```python
from build123d import *

# Parameters (mm, degrees)
ESQUISSE1_W             = 19.5
ESQUISSE1_H             = 1.5
EXTRU_MINCE1_DEPTH      = 96
ESQUISSE2_W             = 1.5
ESQUISSE2_H             = 19.5
EXTRU_MINCE2_DEPTH      = 96
ESQUISSE3_R             = 1.5
ESQUISSE3_W             = 18
ESQUISSE3_H             = 18
ENL_V_MAT_EXTRU_1_DEPTH = 3
ESQUISSE4_R             = 2
ESQUISSE4_R_2           = 1.5
ESQUISSE4_W             = 5
ESQUISSE4_H             = 20
ENL_V_MAT_EXTRU_2_DEPTH = 3
CONG_1_R                = 4


with BuildPart() as part:
    # Esquisse1 → Extru.-Mince1 (new body)
    with BuildSketch(Plane.XY):
        with Locations((0, 0.75)):
            Rectangle(ESQUISSE1_W, ESQUISSE1_H)
    extrude(amount=EXTRU_MINCE1_DEPTH)

    # Esquisse2 → Extru.-Mince2 (add)
    with BuildSketch(Plane(origin=(0, 0, 0), x_dir=(-1, 0, 0), z_dir=(0, 0, -1))):
        with Locations((0, 9.75)):
            Rectangle(ESQUISSE2_W, ESQUISSE2_H)
    extrude(amount=-EXTRU_MINCE2_DEPTH)

    # Esquisse3 → Enlèv. mat.-Extru.1 (cut)
    with BuildSketch(Plane.ZY.offset(0.75)):
        with Locations((48, 16)):
            Circle(ESQUISSE3_R)
        with Locations((9, 10.5)):
            Rectangle(ESQUISSE3_W, ESQUISSE3_H)
        with Locations((87, 10.5)):
            Rectangle(ESQUISSE3_W, ESQUISSE3_H)
    extrude(amount=-ENL_V_MAT_EXTRU_1_DEPTH, mode=Mode.SUBTRACT)

    # Esquisse4 → Enlèv. mat.-Extru.2 (cut)
    with BuildSketch(Plane(origin=(0, 1.5, 0), x_dir=(1, 0, 0), z_dir=(0, 1, 0))):
        with Locations(Location((-0.75, -10, 0), (0, 0, 270))):
            Circle(ESQUISSE4_R)
        with Locations(Location((-0.75, -86, 0), (0, 0, 270))):
            Circle(ESQUISSE4_R)
        with Locations(Location((6.75, -48, 0), (0, 0, 270))):
            Circle(ESQUISSE4_R_2)
        with Locations((7.25, -86)):
            Rectangle(ESQUISSE4_W, ESQUISSE4_H)
    extrude(amount=-ENL_V_MAT_EXTRU_2_DEPTH, mode=Mode.SUBTRACT)

    # Congé1
    cong_1_edges = [part.edges().sort_by_distance(p)[0] for p in [
        (4.75, 0.75, 76),
    ]]
    fillet(cong_1_edges, radius=CONG_1_R)


solid = part.part
```
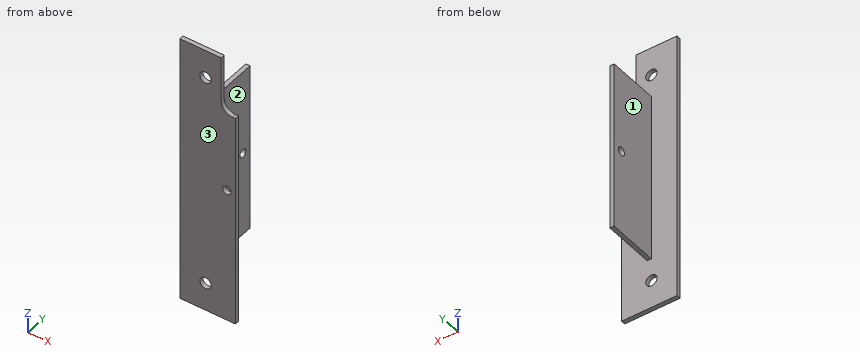
Model file for the job. Use its own axes, mm. Face numbers are marked on the shaded views. A direction names the side the tool comes from. Coordinates: 2 decimals unless noted, no trailing zeros. Write each loop counter-clockwise with the first axis right and the second up, starting at its lowest first coordinate (ties: lowest second). Pieces come first, ordered by that corner, then holes. Notation, with made-up numbers: (62, -23.75) - (77, -23.75) arc R22 ccw to (77, 3.25) - close; hole circle Ø1 at (64, 69.5). An arc over 180 degrees is marked (long way). Use a Markdown table: item, result. Add a question column.
Item 1: Band-saw the part on D-D, the plane z = 38. Write the cut outline in (x, y).
Item 2: 3-axis set-ups, long thin cutter, end or side, ignore diameter. For the marked faces 1, 2 and 3: which of +Z, -Z, +X, -X, +Y, -Y reach the whole face in a straight line?
Item 3: Drill centre lines: line 1 along X through (y, z) = (1.25, 10); line 2 along Y through (x, z) = (0.1, 48); line 3 along Y through (x, z) = (4.75, 72). Where is each one in solid material? Low to high.
Item 4: Band-saw the part on B-B, the plane y = 16. Write the cut outline in (x, z).
Item 5: Drop flat-ended pins along their axis: pin 1 (1 mm diameter, centred on x = -0.5, y = 6.5, fed in from -Z); pin 2 (6 mm diameter, centred on y = 16, z = 41.5, fed in from +X); pin 3 (6.5 mm diameter, centred on x = -0.75, z = 10, fed in from +Y). Give the stop position or say it passes through.
Item 6: Band-saw the part on C-C, the plane z = 48. Write the cut outline in (x, y), and give its area (4 significant figures).
Item 7: Band-saw the part on A-A, the plane z = 86. Write the cut outline in (x, y).
A:
| question | item | result |
|---|---|---|
| 1 | outline | (-9.75, 0) - (9.75, 0) - (9.75, 1.5) - (0.75, 1.5) - (0.75, 19.5) - (-0.75, 19.5) - (-0.75, 1.5) - (-9.75, 1.5) - close |
| 2 | face 1 | +Z, -Z, -X, +Y |
| 2 | face 2 | +Z, -Z, +X, +Y |
| 2 | face 3 | +Z, -Z, +X, -X, -Y |
| 3 | line 1 | x = -9.75 to -2.75, 1.25 to 9.75 |
| 3 | line 2 | y = 0 to 14.5, 17.5 to 19.5 |
| 3 | line 3 | y = 0 to 1.5 |
| 4 | outline | (-0.75, 18) - (0.75, 18) - (0.75, 46.5) - (-0.75, 46.5) - close; (-0.75, 49.5) - (0.75, 49.5) - (0.75, 78) - (-0.75, 78) - close |
| 5 | pin 1 | stops at z = 18 |
| 5 | pin 2 | stops at x = 0.75 |
| 5 | pin 3 | stops at y = 1.5 |
| 6 | outline | (-9.75, 0) - (5.25, 0) - (5.25, 1.5) - (0.75, 1.5) - (0.75, 14.5) - (-0.75, 14.5) - (-0.75, 1.5) - (-9.75, 1.5) - close; (-0.75, 17.5) - (0.75, 17.5) - (0.75, 19.5) - (-0.75, 19.5) - close; (8.25, 0) - (9.75, 0) - (9.75, 1.5) - (8.25, 1.5) - close |
| 6 | area | 47.25 mm² |
| 7 | outline | (-9.75, 0) - (-2.75, 0) - (-2.75, 1.5) - (-9.75, 1.5) - close; (1.25, 0) - (4.75, 0) - (4.75, 1.5) - (1.25, 1.5) - close |
